Autodesk Inventor part; units mm, degrees
sketch "Boceto1" plane through (0, 0, 0) normal (0, 0, 1) x (1, 0, 0)
  line L0 (-75, 75) -> (75, 75)
  line L1 (75, 75) -> (75, -75)
  line L2 (75, -75) -> (-75, -75)
  line L3 (-75, -75) -> (-75, 75)
  line L4 (-75, 75) -> (75, -75) construction
  line L5 (75, 75) -> (-75, -75) construction
  point P0 (0, 0)
  dimension "d0" = 150
  dimension "d1" = 150
extrude "Extrusión1" add sketch "Boceto1" along normal blind 25.4
sketch "Boceto3" plane through (0, 0, 0) normal (0, 1, 0) x (-1, 0, 0)
  line L0 (-75, 25.4) -> (75, 25.4)
  arc A0 (-15, 25.4) -> (15, 25.4) centre (0, 25.4) ccw
  line L1 (15, 25.4) -> (-15, 25.4)
  point P0 (0, 0)
  dimension "d7" = 15
revolve "Revolución2" cut sketch "Boceto3" angle 360 about axis through (75, 0, 25.4) along (-1, 0, 0)
properties part number "Placa - Bolsillo Esfera Radio 15 mm"
Check sheet for the modelled part. Datum: model origin and axes. Units: mm. Give positions to 0.01 mm unless a question says otherwise; leave off trailing zeros. Write each loop counter-clockwise with the first axis right and the second up, starting at its lowest first coordinate (ties: lowest second). Pieces come first, ordered by that corner, then holes. Notation, with made-up numbers: (51.25, -36.75) -> (88.25, -36.75) arc R26 cw to (88.25, -12.75) -> close; hole circle Ø1 at (-37, -7). An arc over 180 degrees is marked (long way). One line per item, written item: value. Start each with the question number.
Item 1: Material ranges on probe 1 along X at (y, z) = (4, 23); probe 2 along X at (y, z) = (-9.5, 15.5); probe 3 along Y at (x, z) = (-3.5, 13), recorded low to high. Write a range as from..to.
Item 2: Section check A-A on z = 17. Record the cut outline in (x, y).
Item 3: Section check B-B on x = -3.5. Record the cut outline in (y, z).
Results list:
1. probe 1: -75..-14.26, 14.26..75
1. probe 2: -75..-6.06, 6.06..75
1. probe 3: -75..-7.68, 7.68..75
2. outline: (-75, -75) -> (75, -75) -> (75, 75) -> (-75, 75) -> close; hole circle Ø24.85 at (0, 0)
3. outline: (-75, 0) -> (75, 0) -> (75, 25.4) -> (14.59, 25.4) arc R14.59 cw to (-14.59, 25.4) -> (-75, 25.4) -> close
